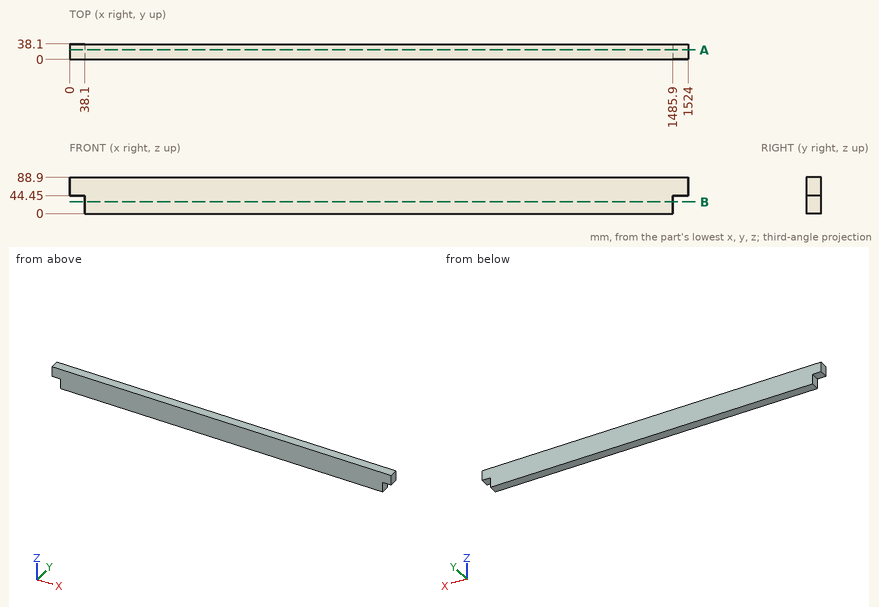
Source: three-view drawing plus pictorial views. Frame: mm from the lowest corner of the part. Give positions to 0.01 mm unless a question says otherwise; leave off trailing zeros. Write each loop counter-clockwise with the first axis right and the second up, starting at its lowest first coordinate (ties: lowest second). Pieces come first, ordered by that corner, then holes.
(1) Cut plane A-A, the plane y = 23.5. Return loops of the section in (x, z).
(2) Ray query, line 1 (X direction, y = 10, z = 24.5). Return the intervals inside material, ascending.
(3) First-contact query: P1, Ø11.5, axis at y = 25.5, z = 16, coming from the -X side; P2, Ø19, axis at x = 1495.5, y = 24.5, coming from the -Z side; P3, Ø12, axis at y = 27.5, z = 14.5, coming from the +X side. Flat tips, straight axial feed; report the tip coordinate or a pass-through.
(4) Cut plane B-B, the plane z = 29. Return loops of the section in (x, y).
Values follow:
1. outline: (0, 44.45) - (38.1, 44.45) - (38.1, 0) - (1485.9, 0) - (1485.9, 44.45) - (1524, 44.45) - (1524, 88.9) - (0, 88.9) - close
2. line 1: x = 38.1 to 1485.9
3. P1: stops at x = 38.1
3. P2: stops at z = 44.45
3. P3: stops at x = 1485.9
4. outline: (38.1, 0) - (1485.9, 0) - (1485.9, 38.1) - (38.1, 38.1) - close
